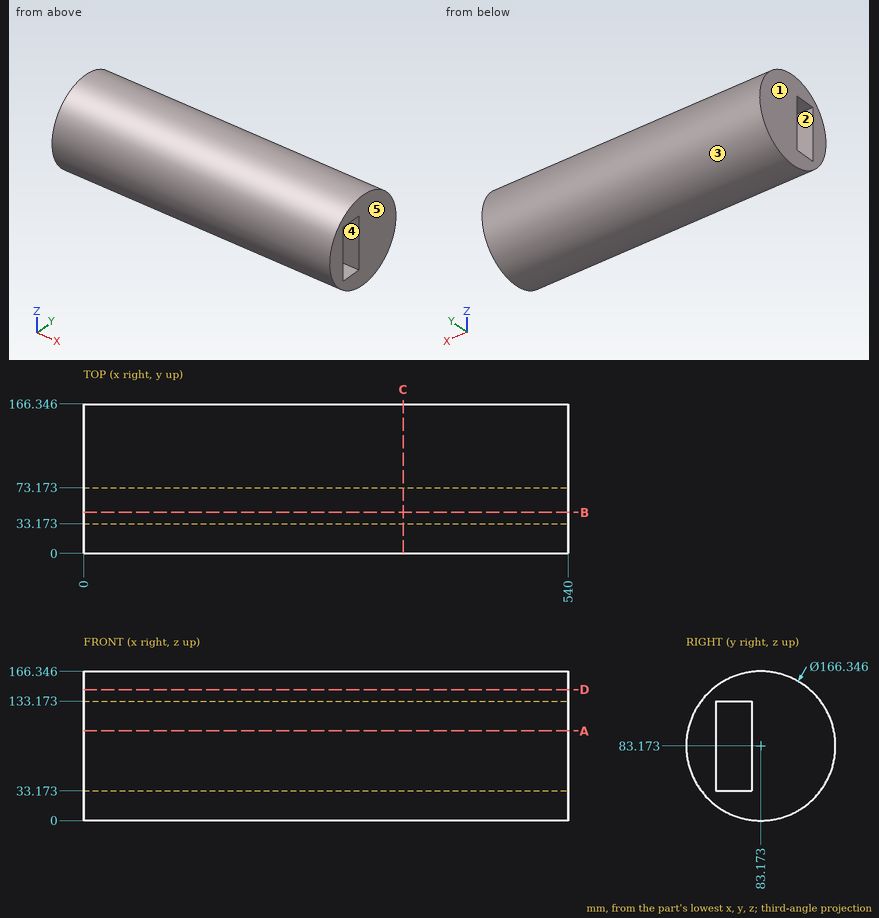
Answer from the drawing. Dimensions are ordinates in mm from the lowest x, y and z of the part. A direction names the side the tool comes from. Give positions to 0.01 mm unless a question says otherwise; leave off trailing zeros. Write each loop counter-clockwise with the first axis right and the second up, starting at its lowest first coordinate (ties: lowest second). Pieces come first, ordered by that corner, then holes.
1) Section B-B (y = 45.5) is taken. Write down the section's boundary in (x, z) (1 decimal), and give its area (3 significant figures).
2) Find the intervals of material crossed by L1, parallel to Y at x = 128, z = 119; L2, parallel to Z at x = 436.5, y = 48; L3, parallel to Y at x = 176.5, z = 98, in increasing order.
3) Section D-D (z = 146) is taken. Write down the section's boundary in (x, y) (1 decimal).
4) Given P1, Ø12, axis at x = 246.5, y = 53, coming from the -Z side; P2, Ø1.5, axis at x = 254.5, z = 21.5, coming from the -Y side; P3, Ø1.5, axis at x = 118, y = 99, coming from the +Z side; P4, Ø8, axis at y = 45, z = 133, coming from the +X side, each flat-ended and moving along its own axis, determine where each tip first touches the part or whether it passes through.
5) A tool of negligible diameter and unlimited length cuts with its end or side. For the marked faces 4 and 5, from which of +Z, -Z, +X, -X, +Y, -Y can it reach the whole face along a straight path? Write none if from no direction.
6) Section A-A (z = 100) is taken. Write down the section's boundary in (x, y), and give its area (3 significant figures).
7) Section C-C (x = 356) is taken. Write down the section's boundary in (y, z), and give its area (3 significant figures).
8) For a pull along Z with two mould halves and no side action, classify the marked faces 1, 2 and 3 as pulls with the +Z half, pulls with the -Z half, needs draft (parallel to the pull), parting line crosses it, or undercut.
Response:
1. outline: (0, 9) - (540, 9) - (540, 33.2) - (0, 33.2) - close; (0, 133.2) - (540, 133.2) - (540, 157.3) - (0, 157.3) - close
1. area: 26,100 mm2
2. L1: y = 8.11 to 33.17, 73.17 to 158.23
2. L2: z = 7.8 to 33.17, 133.17 to 158.54
2. L3: y = 1.33 to 33.17, 73.17 to 165.01
3. outline: (0, 28.7) - (540, 28.7) - (540, 137.7) - (0, 137.7) - close
4. P1: stops at z = 3.59
4. P2: stops at y = 26.55
4. P3: stops at z = 164.97
4. P4: stops at x = 540
5. face 4: +X, -X
5. face 5: +Z, -Z, +X, +Y, -Y
6. outline: (0, 1.72) - (540, 1.72) - (540, 33.17) - (0, 33.17) - close; (0, 73.17) - (540, 73.17) - (540, 164.63) - (0, 164.63) - close
6. area: 66,400 mm2
7. outline: circle Ø166.35 at (83.17, 83.17); hole (33.17, 33.17) - (73.17, 33.17) - (73.17, 133.17) - (33.17, 133.17) - close
7. area: 17,700 mm2
8. face 1: needs draft
8. face 2: undercut
8. face 3: parting line crosses it
